Work out the finished part from the listing and answer in its coordinate system (mm). Coordinates: 2 decimals unless noted, no trailing zeros. Order: outer loops, then holes, each group sorted by start corner. A loop starts at its lowest first (then second) coordinate and runs counter-clockwise, first axis right, second up.
1. Determine the mould class of faces 1 (the flat face through (0, -61.25, 3)), 2 (the cylindrical face through (-13.36, 44.91, 2.96)), 3 (the flat face through (31, -1, 3)) for opening direction X: +X half, -X half, draft (parallel to the pull), parting line (faces both ways), or undercut.
2. Find the intervals of material crossed by probe 1 along Y at (x, z) = (-12.5, 3.8); probe 2 along Y at (x, z) = (-25.5, 2.55); probe 3 along X at (y, z) = (3, 5.3), in increasing order.
3. The part is cut by section C-C, the plane z = 1.2. Count the separate pieces of the cut face and the enclosed holes in it, then the cut area to 3 significant figures.
4. A flat-ended cylindrical pin translates along its axis: pin 1 Ø4 at (x, y) = (-12.8, 47.45) entering from -Z. Find the tip coordinate at first contact, or state that the pin passes through.
5. The part is cut by section A-A, the plane y = 47.45. Give the vertices of the cut face in (x, z), then the cut area to 3 significant figures.
6. The part is cut by section B-B, the plane x = -12.8. Give the vertices of the cut face in (y, z), then the cut area to 3 significant figures.
```python
from build123d import *

# Parameters (mm, degrees)
SKETCH_1_W      = 62
SKETCH_1_H      = 122.5
SKETCH_1_R      = 2
SKETCH_1_R_2    = 2.6
EXTRUDE_1_DEPTH = 6


with BuildPart() as part:
    # 草图1 → 凸台-拉伸1 (new body)
    with BuildSketch(Plane.XY):
        Rectangle(SKETCH_1_W, SKETCH_1_H)
        with Locations((-25.5, 35.45)):
            Circle(SKETCH_1_R, mode=Mode.SUBTRACT)
        with Locations((-25.5, 14.45)):
            Circle(SKETCH_1_R, mode=Mode.SUBTRACT)
        with Locations(Location((25.5, 14.45, 0), (0, 0, 180))):
            Circle(SKETCH_1_R, mode=Mode.SUBTRACT)
        with Locations(Location((25.5, 35.45, 0), (0, 0, 180))):
            Circle(SKETCH_1_R, mode=Mode.SUBTRACT)
        with Locations((-12.8, 47.45)):
            Circle(SKETCH_1_R_2, mode=Mode.SUBTRACT)
        with Locations(Location((12.8, 47.45, 0), (0, 0, 180))):
            Circle(SKETCH_1_R_2, mode=Mode.SUBTRACT)
        with Locations((12.8, 2.45)):
            Circle(SKETCH_1_R_2, mode=Mode.SUBTRACT)
        with Locations(Location((-12.8, 2.45, 0), (0, 0, 180))):
            Circle(SKETCH_1_R_2, mode=Mode.SUBTRACT)
    extrude(amount=EXTRUDE_1_DEPTH)


solid = part.part
```
Geometry says:
1. face 1: draft
1. face 2: undercut
1. face 3: +X half
2. probe 1: y = -61.25 to -0.13, 5.03 to 44.87, 50.03 to 61.25
2. probe 2: y = -61.25 to 12.45, 16.45 to 33.45, 37.45 to 61.25
2. probe 3: x = -31 to -15.34, -10.26 to 10.26, 15.34 to 31
3. separate pieces: 1
3. enclosed holes: 8
3. area: 7,460 mm2
4. pin 1: passes through
5. outline: (-31, 0) - (-15.4, 0) - (-15.4, 6) - (-31, 6) - close; (-10.2, 0) - (10.2, 0) - (10.2, 6) - (-10.2, 6) - close; (15.4, 0) - (31, 0) - (31, 6) - (15.4, 6) - close
5. area: 310 mm2
6. outline: (-61.25, 0) - (-0.15, 0) - (-0.15, 6) - (-61.25, 6) - close; (5.05, 0) - (44.85, 0) - (44.85, 6) - (5.05, 6) - close; (50.05, 0) - (61.25, 0) - (61.25, 6) - (50.05, 6) - close
6. area: 673 mm2
